The drawing under review shows one solid part. Ordinate dimensions are in mm from its lowest x, y, z. A direction names the side the tool comes from. Give positions to 0.01 mm unless a question says otherwise; leave off trailing zeros. Write each loop counter-clockwise with the first axis right and the second up, starting at its lowest first coordinate (ties: lowest second). Pieces come first, ordered by that corner, then holes.
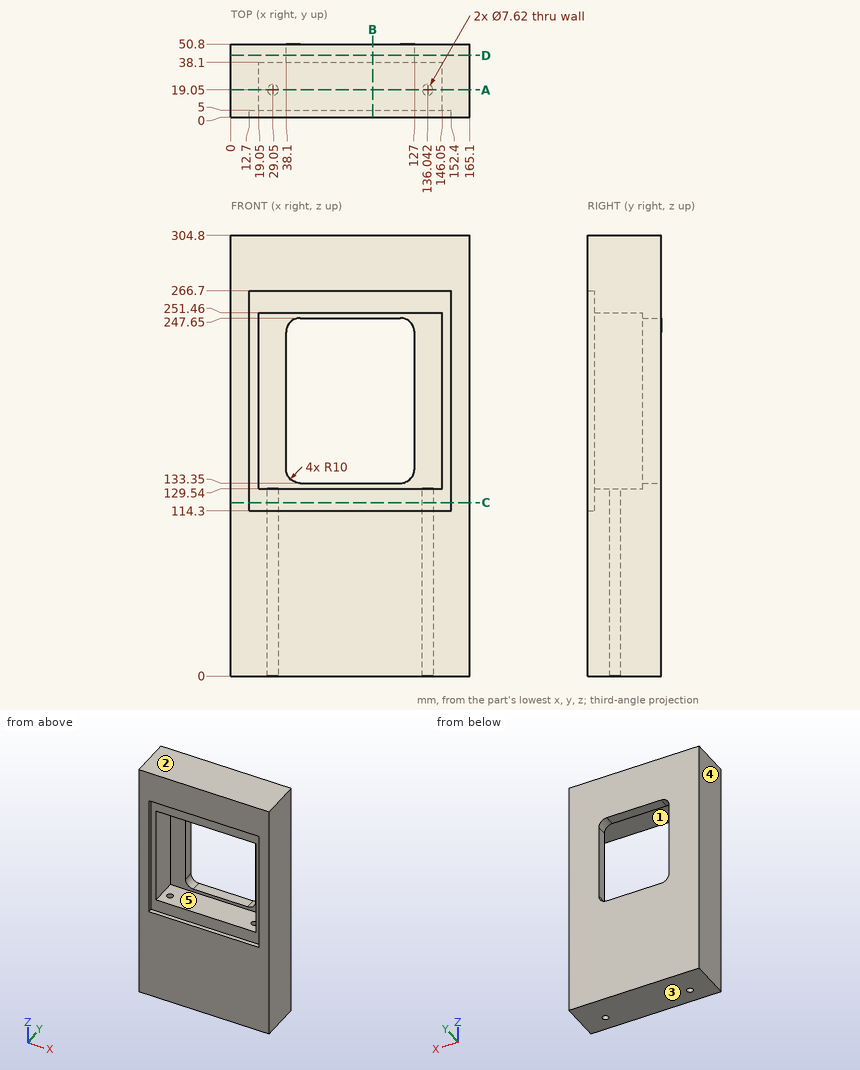
1) Insertion check: pin 1 (10 mm diameter, centred on x = 123, z = 156.5, fed in from -Y); pin 2 (4.5 mm diameter, centred on x = 136.04, y = 19.05, fed in from -Z). Each pin has a flat end and moves straight along its axis. Give the tip position at first contact, or say it passes through.
2) Tool access review of the marked faces 1 and 2: name each direction out of +Z, -Z, +X, -X, +Y, -Y from which nothing blocks a thin tool from reaching the whole face with its end or side.
3) The part is to be moulded in two halves that separate along Z. For the marked faces 3, 4 and 5, say which applies: +Z half, -Z half, draft (parallel to the pull), parting line (faces both ways), or undercut.
4) Consider section A-A, the plane y = 19.05. Give the boundary of the cut face in (x, z), then the cut area to 3 significant figures.
5) To check wall thickness, follow probe 1 along X at (y, z) = (19, 55); probe 2 along X at (y, z) = (15.5, 157.5); probe 3 along Z at (x, y) = (33.5, 28). State the ranges of each line that lie inside material, in increasing order.
6) Consider section C-C, the plane z = 120. Give the boundary of the cut face in (x, y), then the cut area to 3 significant figures.
7) Consider section D-D, the plane y = 43. Give the boundary of the cut face in (x, z).
8) Consider section B-B, the plane x = 98. Give the boundary of the cut face in (y, z).
Answer block:
1. pin 1: stops at y = 38.1
1. pin 2: stops at z = 251.46
2. face 1: -Y
2. face 2: +Z, +X, -X, +Y, -Y
3. face 3: -Z half
3. face 4: draft
3. face 5: undercut
4. outline: (0, 0) - (25.24, 0) - (25.24, 129.54) - (19.05, 129.54) - (19.05, 251.46) - (146.05, 251.46) - (146.05, 129.54) - (139.85, 129.54) - (139.85, 0) - (165.1, 0) - (165.1, 304.8) - (0, 304.8) - close; (32.86, 0) - (132.23, 0) - (132.23, 129.54) - (32.86, 129.54) - close
4. area: 32,900 mm2
5. probe 1: x = 0 to 25.24, 32.86 to 132.23, 139.85 to 165.1
5. probe 2: x = 0 to 19.05, 146.05 to 165.1
5. probe 3: z = 0 to 129.54, 251.46 to 304.8
6. outline: (0, 0) - (12.7, 0) - (12.7, 5) - (152.4, 5) - (152.4, 0) - (165.1, 0) - (165.1, 50.8) - (0, 50.8) - close; hole circle Ø7.62 at (29.05, 19.05); hole circle Ø7.62 at (136.04, 19.05)
6. area: 7,600 mm2
7. outline: (0, 0) - (165.1, 0) - (165.1, 304.8) - (0, 304.8) - close; hole (38.1, 143.35) arc R10 ccw to (48.1, 133.35) - (117, 133.35) arc R10 ccw to (127, 143.35) - (127, 237.65) arc R10 ccw to (117, 247.65) - (48.1, 247.65) arc R10 ccw to (38.1, 237.65) - close
8. outline: (0, 0) - (50.8, 0) - (50.8, 133.35) - (38.1, 133.35) - (38.1, 129.54) - (5, 129.54) - (5, 114.3) - (0, 114.3) - close; (0, 266.7) - (5, 266.7) - (5, 251.46) - (38.1, 251.46) - (38.1, 247.65) - (50.8, 247.65) - (50.8, 304.8) - (0, 304.8) - close
